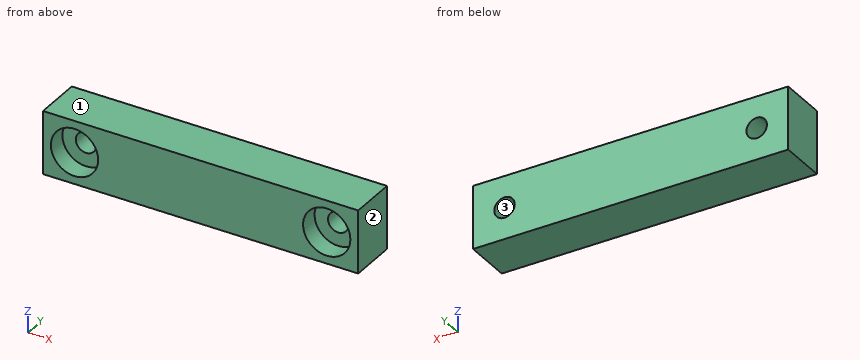
```python
from build123d import *

# Parameters (mm, degrees)
SKETCH1_W           = 100
SKETCH1_H           = 20
BOSS_EXTRUDE1_DEPTH = 15
SKETCH2_R           = 7.5
CUT_EXTRUDE1_DEPTH  = 6
SKETCH3_R           = 3.25
CUT_EXTRUDE2_DEPTH  = 103.376755174


with BuildPart() as part:
    # Sketch1 → Boss-Extrude1 (new body)
    with BuildSketch(Plane(origin=(0, 0, 0), x_dir=(1, 0, 0), z_dir=(0, 1, 0))):
        with Locations((50, 10)):
            Rectangle(SKETCH1_W, SKETCH1_H)
    extrude(amount=BOSS_EXTRUDE1_DEPTH)

    # Sketch2 → Cut-Extrude1 (cut)
    with BuildSketch(Plane.XZ):
        with Locations(Location((10, -10, 0), (0, 0, 270))):
            Circle(SKETCH2_R)
        with Locations(Location((90, -10, 0), (0, 0, 270))):
            Circle(SKETCH2_R)
    extrude(amount=-CUT_EXTRUDE1_DEPTH, mode=Mode.SUBTRACT)

    # Sketch3 → Cut-Extrude2 (cut, through all)
    with BuildSketch(Plane.XZ.offset(-6)):
        with Locations(Location((10, -10, 0), (0, 0, 270))):
            Circle(SKETCH3_R)
        with Locations(Location((90, -10, 0), (0, 0, 270))):
            Circle(SKETCH3_R)
    extrude(amount=-CUT_EXTRUDE2_DEPTH, mode=Mode.SUBTRACT)


solid = part.part
```
Geometry check sheet. Reference: the model listing, model coordinates, mm. Face numbers are marked on the shaded views. Coordinates: 2 decimals unless noted, no trailing zeros. Order: outer loops, then holes, each group sorted by start corner. A loop starts at its lowest first (then second) coordinate and runs counter-clockwise, first axis right, second up. Notation, with made-up numbers: (-19.5, 46) - (3.5, 46) arc R19 ccw to (3.5, 62) - close; hole circle Ø9 at (48.25, -29.75). An arc over 180 degrees is marked (long way). Answer as a JSON object with one key per item and string values. Group by question number.
Item 1: Draft check along X on the marked faces 1, 2 and 3. Enter one of: +X half, -X half, draft (parallel to the pull), parting line (faces both ways), or undercut.
Item 2: Sectioned sample at A-A, the plane x = 10. Record the cut outline in (y, z).
Item 3: Scan lines: probe 1 along X at (y, z) = (2.2, -10); probe 2 along X at (y, z) = (9.25, -10); probe 3 along Z at (x, y) = (92, 9.5). Record each from-to range of solid material in increasing order.
Item 4: Sectioned sample at C-C, the plane z = -10.25. Record the cut outline in (x, y), and give its area (3 significant figures).
Item 5: Sectioned sample at B-B, the plane y = 9.5. Record the cut outline in (x, z).
Item 6: Depth check by flat-ended pin: pin 1 Ø4.5 at (x, z) = (91, -12.5) entering from -Y; pin 2 Ø6 at (x, z) = (10, -10) entering from -Y. Enter the tip coordinate at first touch or a pass-through.
Item 7: Sectioned sample at D-D, the plane z = -4. Record the cut outline in (x, y), and give its area (3 significant figures).
Resolved:
{
 "1": {"face 1": "draft", "face 2": "+X half", "face 3": "undercut"},
 "2": {"outline": "(0, -20) - (15, -20) - (15, -13.25) - (6, -13.25) - (6, -17.5) - (0, -17.5) - close; (0, -2.5) - (6, -2.5) - (6, -6.75) - (15, -6.75) - (15, 0) - (0, 0) - close"},
 "3": {"probe 1": "0 to 2.5, 17.5 to 82.5, 97.5 to 100", "probe 2": "0 to 6.75, 13.25 to 86.75, 93.25 to 100", "probe 3": "-20 to -12.56, -7.44 to 0"},
 "4": {"outline": "(0, 0) - (2.5, 0) - (2.5, 6) - (6.76, 6) - (6.76, 15) - (0, 15) - close; (13.24, 6) - (17.5, 6) - (17.5, 0) - (82.5, 0) - (82.5, 6) - (86.76, 6) - (86.76, 15) - (13.24, 15) - close; (93.24, 6) - (97.5, 6) - (97.5, 0) - (100, 0) - (100, 15) - (93.24, 15) - close", "area": "1,200 mm^2"},
 "5": {"outline": "(0, -20) - (100, -20) - (100, 0) - (0, 0) - close; hole circle Ø6.5 at (10, -10); hole circle Ø6.5 at (90, -10)"},
 "6": {"pin 1": "y = 6", "pin 2": "through"},
 "7": {"outline": "(0, 0) - (5.5, 0) - (5.5, 6) - (14.5, 6) - (14.5, 0) - (85.5, 0) - (85.5, 6) - (94.5, 6) - (94.5, 0) - (100, 0) - (100, 15) - (0, 15) - close", "area": "1,390 mm^2"}
}
